Check sheet for the modelled part. Datum: model origin and axes. Units: mm. Face numbers are marked on the shaded views. A direction names the side the tool comes from. Coordinates: 2 decimals unless noted, no trailing zeros. Loops run counter-clockwise (first coordinate to the right, second up) from the corner with the lowest first, then second, coordinate; pieces in that order, holes last. Notation, with made-up numbers: (19, -39) -> (67, -39) arc R17 ccw to (67, -8) -> close; hole circle Ø6 at (-13, 49.5). An arc over 180 degrees is marked (long way). Use CSV: the item, a comma, the result in double quotes.
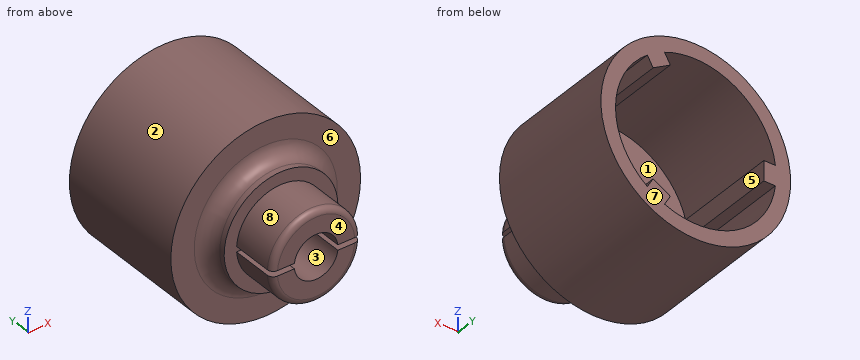
```python
from build123d import *

# Parameters (mm, degrees)
SKETCH1_R           = 32.5
BOSS_EXTRUDE1_DEPTH = 46.3
SKETCH2_R           = 27.5
CUT_EXTRUDE1_DEPTH  = 40
SKETCH3_R           = 19.5
BOSS_EXTRUDE2_DEPTH = 7
SKETCH4_R           = 15.25
BOSS_EXTRUDE3_DEPTH = 16
FILLET1_R           = 5
SKETCH7_W           = 66.193685288
SKETCH7_H           = 1.806726502
CUT_EXTRUDE2_DEPTH  = 16
FILLET2_R           = 2
SKETCH9_W           = 9
SKETCH9_H           = 6.8
BOSS_EXTRUDE4_DEPTH = 40
SKETCH8_R           = 7.5
CUT_EXTRUDE3_DEPTH  = 61.930288035
CIRPATTERN1_COUNT   = 3


with BuildPart() as part:
    # Sketch1 → Boss-Extrude1 (new body)
    with BuildSketch(Plane(origin=(0, 0, 0), x_dir=(1, 0, 0), z_dir=(0, 1, 0))):
        with Locations(Location((0, 0, 0), (0, 0, 270))):
            Circle(SKETCH1_R)
    extrude(amount=BOSS_EXTRUDE1_DEPTH)

    # Sketch2 → Cut-Extrude1 (cut)
    with BuildSketch(Plane(origin=(0, 46.3, 0), x_dir=(1, 0, 0), z_dir=(0, 1, 0))):
        with Locations(Location((0, 0, 0), (0, 0, 270))):
            Circle(SKETCH2_R)
    extrude(amount=-CUT_EXTRUDE1_DEPTH, mode=Mode.SUBTRACT)

    # Sketch3 → Boss-Extrude2 (add)
    with BuildSketch(Plane.XZ):
        with Locations(Location((0, 0, 0), (0, 0, 270))):
            Circle(SKETCH3_R)
    extrude(amount=BOSS_EXTRUDE2_DEPTH)

    # Sketch4 → Boss-Extrude3 (add)
    with BuildSketch(Plane.XZ.offset(7)):
        with Locations(Location((0, 0, 0), (0, 0, 270))):
            Circle(SKETCH4_R)
    extrude(amount=BOSS_EXTRUDE3_DEPTH)

    # Fillet1
    fillet1_edges = [part.edges().sort_by_distance(p)[0] for p in [
        (0, 0, 19.5),
    ]]
    fillet(fillet1_edges, radius=FILLET1_R)

    # Sketch7 → Cut-Extrude2 (cut)
    with BuildSketch(Plane.XZ.offset(23)):
        Rectangle(SKETCH7_W, SKETCH7_H)
    extrude(amount=-CUT_EXTRUDE2_DEPTH, mode=Mode.SUBTRACT)

    # Fillet2
    fillet2_edges = [part.edges().sort_by_distance(p)[0] for p in [
        (0, -23, 15.25),
        (0, -23, -15.25),
    ]]
    fillet(fillet2_edges, radius=FILLET2_R)

    # Sketch9 → Boss-Extrude4 (add)
    with BuildSketch(Plane(origin=(0, 46.3, 0), x_dir=(1, 0, 0), z_dir=(0, 1, 0))):
        with Locations((-27.821664561, 0)):
            Rectangle(SKETCH9_W, SKETCH9_H)
    boss_extrude4 = extrude(amount=-BOSS_EXTRUDE4_DEPTH)

    # Sketch8 → Cut-Extrude3 (cut, through all)
    with BuildSketch(Plane(origin=(0, 6.3, 0), x_dir=(1, 0, 0), z_dir=(0, 1, 0))):
        with Locations(Location((0, 0, 0), (0, 0, 270))):
            Circle(SKETCH8_R)
    extrude(amount=-CUT_EXTRUDE3_DEPTH, mode=Mode.SUBTRACT)

    # CirPattern1: Boss-Extrude4 ×3 about axis
    cirpattern1_axis = Axis((0, 0, 0), (0, 1, 0))
    for i in range(1, CIRPATTERN1_COUNT):
        add(boss_extrude4.rotate(cirpattern1_axis, i * 360 / CIRPATTERN1_COUNT))


solid = part.part
```
1) Cross-section at B-B on y = 37.5. Record the boundary of the cut face in (x, z).
Answer below:
outline,"circle Ø65 at (0, 0); hole (-27.29, -3.4) arc R27.5 ccw to (10.7, -25.33) -> (8.72, -21.9) -> (14.61, -18.5) -> (16.59, -21.93) arc R27.5 ccw to (16.59, 21.93) -> (14.61, 18.5) -> (8.72, 21.9) -> (10.7, 25.33) arc R27.5 ccw to (-27.29, 3.4) -> (-23.32, 3.4) -> (-23.32, -3.4) -> close"
2) Draft check along Z on the marked faces 1, 2, 3 and 4. Enter one of: released by +Z, released by -Z, zero draft, split by the parting line, or undercut.
Answer below:
face 1,"undercut"
face 2,"split by the parting line"
face 3,"undercut"
face 4,"zero draft"
3) Cross-section at C-C on y = -1.5. Record the boundary of the cut face in (x, z).
Answer below:
outline,"circle Ø41.86 at (0, 0); hole circle Ø15 at (0, 0)"
4) Access from +Z, -Z, +X, -X, +Y, -Y to the whole of each face (thin tool, end or side, straight path). Record for the marked faces 5, 6, 7 and 8.
Answer below:
face 5,"+Y"
face 6,"-Y"
face 7,"+Z, -Z, +X, -X, +Y"
face 8,"+Z, -Y"
5) Go/stop test with flat-tipped pins: pin 1 Ø2.5 at (x, y) = (-12.5, -18) entering from +Z; pin 2 Ø6 at (x, y) = (13, -13) entering from -Z; pin 3 Ø2 at (x, z) = (18, 8.5) entering from -Y; pin 4 Ø12 at (x, z) = (0, 0) entering from -Y. Record where each tip stops, or that it passes through.
Answer below:
pin 1,"stops at z = 10.3"
pin 2,"stops at z = -11.51"
pin 3,"stops at y = -7"
pin 4,"passes through"
6) Thickness scan on line 1 along X through (y, z) = (0.5, 0); line 2 along Z through (x, y) = (0, -17); line 3 along X through (y, z) = (-4.5, 0). Record the ranges inside material, lowest first. Write a range as from..to.
Answer below:
line 1,"x = -32.5..-7.5, 7.5..32.5"
line 2,"z = -15.25..-7.5, 7.5..15.25"
line 3,"x = -19.53..-7.5, 7.5..19.53"
7) Cross-section at A-A on x = 0. Record the boundary of the cut face in (y, z), and give its area (3 significant figures).
Answer below:
outline,"(-23, -13.25) arc R2 ccw to (-21, -15.25) -> (-7, -15.25) -> (-7, -19.5) -> (-5, -19.5) arc R5 cw to (0, -24.5) -> (0, -32.5) -> (46.3, -32.5) -> (46.3, -27.5) -> (6.3, -27.5) -> (6.3, -7.5) -> (-23, -7.5) -> close; (-23, 7.5) -> (6.3, 7.5) -> (6.3, 27.5) -> (46.3, 27.5) -> (46.3, 32.5) -> (0, 32.5) -> (0, 24.5) arc R5 cw to (-5, 19.5) -> (-7, 19.5) -> (-7, 15.25) -> (-21, 15.25) arc R2 ccw to (-23, 13.25) -> close"
area,"1,140 mm²"
